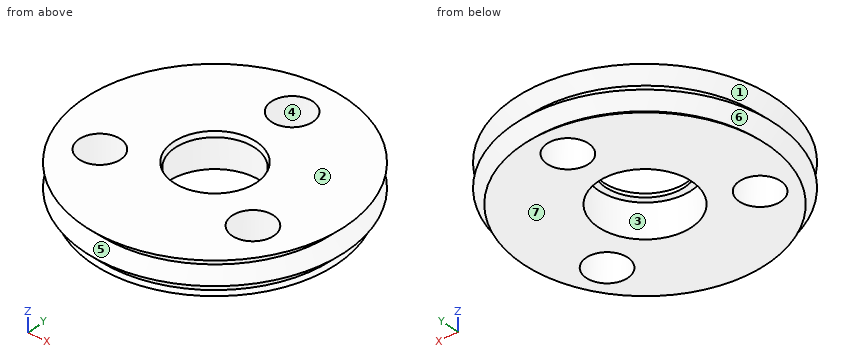
```python
from build123d import *

# Parameters (mm, degrees)
SKETCH019_W    = 10
SKETCH019_H    = 2.7812096768
SKETCH005_W    = 10
SKETCH005_H    = 2.2955317108
CYLINDER_R     = 1.4
CYLINDER_DEPTH = 10
ARRAY001_COUNT = 3
SKETCH018_W    = 3.15
SKETCH018_H    = 2.3
SKETCH002_W    = 5
SKETCH002_H    = 6.8
ARRAY_Z_COUNT  = 6
ARRAY_Z_PITCH  = 1.6


with BuildPart() as obj1:
    # Sketch019 → Revolution008 (revolve)
    with BuildSketch(Plane.XZ):
        with Locations((5, 3.1861365492)):
            Rectangle(SKETCH019_W, SKETCH019_H)
    revolve(axis=Axis((0, 0, 0), (0, 0, 1)))


with BuildPart() as clone_of_lowerdomain001:
    # Sketch005 → Revolution004 (revolve)
    with BuildSketch(Plane.XZ):
        with Locations((5, 0.6477658554)):
            Rectangle(SKETCH005_W, SKETCH005_H)
    revolve(axis=Axis((0, 0, 0), (0, 0, 1)))


with BuildPart() as boltholes:
    # Cylinder → Cylinder (new body)
    with BuildSketch(Plane(origin=(0, 6, -1), x_dir=(1, 0, 0), z_dir=(0, 0, 1))):
        Circle(CYLINDER_R)
    extrude(amount=CYLINDER_DEPTH)

    # Array001: BoltHoles ×3 about axis
    array001_axis = Axis((0, 0, 0), (0, 0, 1))


with BuildPart() as boltholes_1:
    add(boltholes.part)
    for i in range(1, ARRAY001_COUNT):
        add(boltholes.part.rotate(array001_axis, i * 360 / ARRAY001_COUNT))


with BuildPart() as obj2:
    # Sketch018 → Revolution007 (revolve)
    with BuildSketch(Plane.XZ):
        with Locations((1.575, 5.7267413876)):
            Rectangle(SKETCH018_W, SKETCH018_H)
    revolve(axis=Axis((0, 0, 0), (0, 0, 1)))


with BuildPart() as obj3:
    # Sketch007 → Revolution006 (revolve)
    with BuildSketch(Plane.XZ):
        with BuildLine():
            ThreePointArc((1.5, 1.7955317108), (0.867020761, 2.4322916436), (0, 2.6655317108))
            Line((0, 2.6655317108), (0, 0.7955317108))
            Line((0, 0.7955317108), (1.5, 0.7955317108))
            Line((1.5, 1.7955317108), (1.5, 0.7955317108))
        make_face()
    revolve(axis=Axis((0, 0, 0), (0, 0, 1)))


with BuildPart() as obj4:
    # Sketch002 → Revolution002 (revolve)
    with BuildSketch(Plane.XZ):
        with Locations((7.5, 3.8)):
            Rectangle(SKETCH002_W, SKETCH002_H)
    revolve(axis=Axis((0, 0, 0), (0, 0, 1)))


with BuildPart() as innergroovetool:
    # Sketch001 → Revolution001 (revolve)
    with BuildSketch(Plane.XZ):
        Polygon((4, 8), (4, 6.4), (8, 6.4), (8.8, 7.2), (8, 8), align=None)
    revolve(axis=Axis((0, 0, 0), (0, 0, 1)))

    # Array Z: InnerGrooveTool ×6


with BuildPart() as innergroovetool_1:
    add(innergroovetool.part)
    with Locations(*[(0, 0, -i * ARRAY_Z_PITCH) for i in range(1, ARRAY_Z_COUNT)]):
        add(innergroovetool.part)

    # Common: intersect obj4
    add(obj4.part, mode=Mode.INTERSECT)


with BuildPart() as obj5:
    # Sketch → Revolution (revolve)
    with BuildSketch(Plane.XZ):
        Polygon((1.2, 0.4), (8, 0.4), (8, 7.2), (2.8, 7.2), (1.2, 2.2), align=None)
    revolve(axis=Axis((0, 0, 0), (0, 0, 1)))

    # Fusion001: union InnerGrooveTool
    add(innergroovetool_1.part)

    # Cut: cut obj3
    add(obj3.part, mode=Mode.SUBTRACT)

    # Cut003: cut obj2
    add(obj2.part, mode=Mode.SUBTRACT)

    # Cut001: cut BoltHoles
    add(boltholes_1.part, mode=Mode.SUBTRACT)

    # Cut002: cut Clone of LowerDomain001
    add(clone_of_lowerdomain001.part, mode=Mode.SUBTRACT)

    # Cut004: cut obj1
    add(obj1.part, mode=Mode.SUBTRACT)


solid = obj5.part
```
Could you check a few things on this model? Use its own coordinates, in mm. Face numbers are marked on the shaded views. A direction names the side the tool comes from. Give positions to 0.01 mm unless a question says otherwise; leave off trailing zeros. Loops run counter-clockwise (first coordinate to the right, second up) from the corner with the lowest first, then second, coordinate; pieces in that order, holes last. Notation, with made-up numbers: (34.25, 74) - (93.25, 74) arc R17 ccw to (93.25, 90) - close; hole circle Ø3 at (-37, 13). An arc over 180 degrees is marked (long way). Answer in a Markdown table with one row per item. Add a question column.
Q1. Please list where these lines run through material, in increasing order: L1, parallel to Y at x = 0, z = 5.75; L2, parallel to Y at x = -1, z = 7; L3, parallel to X at y = -3.75, z = 5.4. Write a range as from..to.
Q2. Which directions (+Z, -Z, +X, -X, +Y, -Y) give clear straight access to the entire face, cutting with the end or side of a thin tool? Please do the marked faces 1, 2 and 3.
Q3. We'd pull the mould along Z, two halves only. Please class the marked faces 4, 5, 6 and 7: +Z half, -Z half, draft (parallel to the pull), parting line (faces both ways), or undercut.
Q4. For pin 1 (5 mm diameter, centred on x = 0, y = 0, fed in from -Z); pin 2 (1 mm diameter, centred on y = -1.5, z = 5.5, fed in from -X), each with a flat end and sliding along its axis, tell me the tip position at first contact or that it passes through.
Q5. If we section it at A-A (x = 0): List the corners of the cut face in (y, z) for me.
The answers:
| question | item | result |
|---|---|---|
| 1 | L1 | y = -8.65..-3.15, 3.15..4.6, 7.4..8.65 |
| 1 | L2 | y = -8.54..-2.55, 2.55..5.02, 6.98..8.54 |
| 1 | L3 | x = -7.74..-6.38, -4.01..4.01, 6.38..7.74 |
| 2 | face 1 | none |
| 2 | face 2 | +Z, +X, -X, +Y, -Y |
| 2 | face 3 | -Z |
| 3 | face 4 | draft |
| 3 | face 5 | undercut |
| 3 | face 6 | undercut |
| 3 | face 7 | -Z half |
| 4 | pin 1 | passes through |
| 4 | pin 2 | stops at x = -8.74 |
| 5 | outline | (-8.8, 5.6) - (-8, 4.8) - (-8.22, 4.58) - (-3.15, 4.58) - (-3.15, 6.88) - (-2.7, 6.88) - (-2.8, 7.2) - (-8.8, 7.2) - (-8, 6.4) - close; (2.7, 6.88) - (3.15, 6.88) - (3.15, 4.58) - (4.6, 4.58) - (4.6, 7.2) - (2.8, 7.2) - close; (7.4, 4.58) - (8.22, 4.58) - (8, 4.8) - (8.8, 5.6) - (8, 6.4) - (8.8, 7.2) - (7.4, 7.2) - close |
